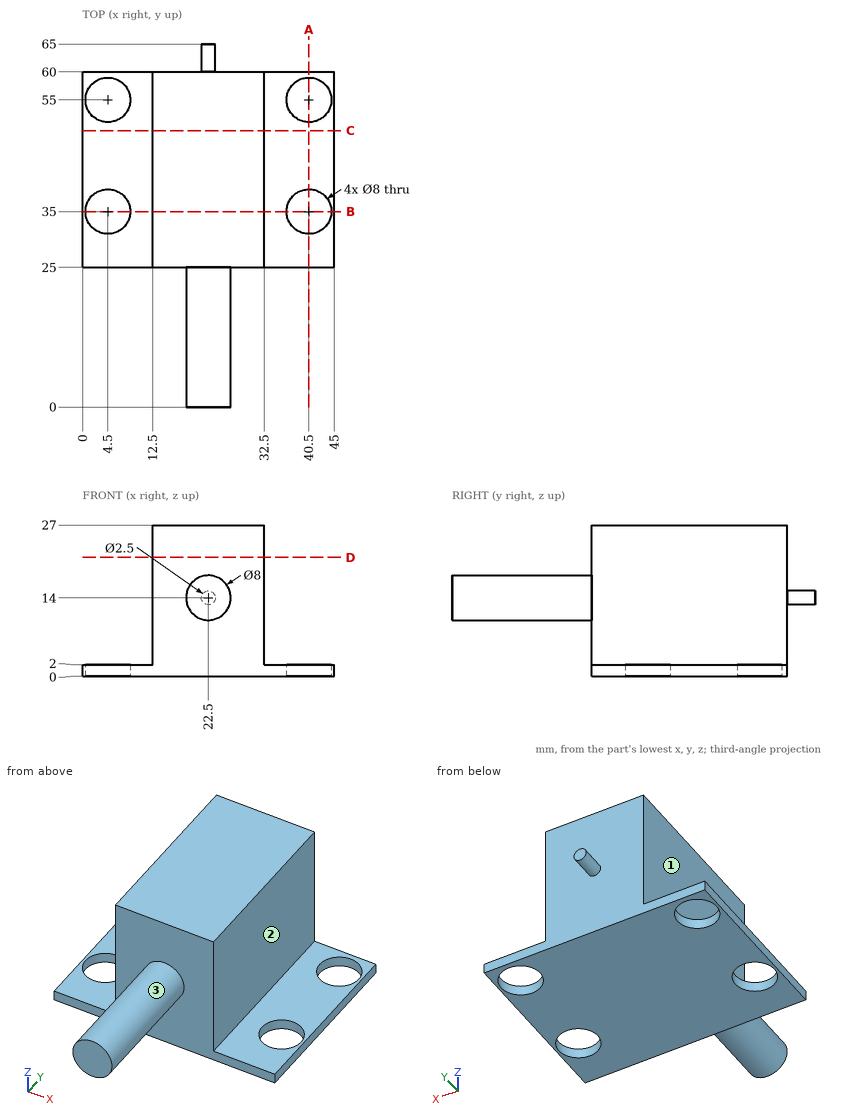
Print and shaded views of the part. All mm, measured from the part's lowest x, y and z. A direction names the side the tool comes from. Give positions to 0.01 mm unless a question says otherwise; leave off trailing zeros. Loops run counter-clockwise (first coordinate to the right, second up) from the corner with the lowest first, then second, coordinate; pieces in that order, holes last.
1) Wall check: line 1 (Y direction, x = 40.5, z = 0.5); line 2 (Y direction, x = 17.5, z = 5.75); line 3 (X direction, y = 39, z = 22.25). Give the ranges that are in metal, low to high.
2) Saw through at D-D (z = 21.25). Write the cut outline in (x, y).
3) Saw through at B-B (y = 35). Write the cut outline in (x, z), plus the area to 3 significant figures.
4) Flat gauge pins, fed straight in: pin 1 Ø1 at (x, z) = (25.5, 16.5) entering from +Y; pin 2 Ø1 at (x, y) = (20, 16.5) entering from +Z; pin 3 Ø1.5 at (x, y) = (17, 8.5) entering from +Z; pin 4 Ø6 at (x, y) = (8.5, 34.5) entering from +Z. Where does each tip first touch, or does it go through?
5) Tool access for the marked faces 1, 2 and 3: list every direction of +Z, -Z, +X, -X, +Y, -Y with a clear straight run to the whole face (end or side of a thin tool).
6) Saw through at C-C (y = 49.5). Write the cut outline in (x, z), plus the area to 3 significant figures.
7) Saw through at A-A (x = 40.5). Write the cut outline in (y, z), plus the area to 3 significant figures.
Answer block:
1. line 1: y = 25 to 31, 39 to 51, 59 to 60
1. line 2: y = 25 to 60
1. line 3: x = 12.5 to 32.5
2. outline: (12.5, 25) - (32.5, 25) - (32.5, 60) - (12.5, 60) - close
3. outline: (0, 0) - (0.5, 0) - (0.5, 2) - (0, 2) - close; (8.5, 0) - (36.5, 0) - (36.5, 2) - (32.5, 2) - (32.5, 27) - (12.5, 27) - (12.5, 2) - (8.5, 2) - close; (44.5, 0) - (45, 0) - (45, 2) - (44.5, 2) - close
3. area: 558 mm2
4. pin 1: stops at y = 60
4. pin 2: stops at z = 17.46
4. pin 3: passes through
4. pin 4: stops at z = 2
5. face 1: +Z, -X, +Y, -Y
5. face 2: +Z, +X, +Y, -Y
5. face 3: -Y
6. outline: (0, 0) - (45, 0) - (45, 2) - (32.5, 2) - (32.5, 27) - (12.5, 27) - (12.5, 2) - (0, 2) - close
6. area: 590 mm2
7. outline: (25, 0) - (31, 0) - (31, 2) - (25, 2) - close; (39, 0) - (51, 0) - (51, 2) - (39, 2) - close; (59, 0) - (60, 0) - (60, 2) - (59, 2) - close
7. area: 38.0 mm2
